The model under review builds one solid part; all positions refer to its coordinate system, in mm. A direction names the side the tool comes from. Round coordinates to 2 decimals unless told otherwise and drop trailing zeros. Write each loop counter-clockwise with the first axis right and the second up, starting at its lowest first coordinate (ties: lowest second). Pieces come first, ordered by that corner, then holes. Notation, with made-up numbers: (5, 73.5) -> (22, 73.5) arc R23 ccw to (22, 103.5) -> close; hole circle Ø2 at (6.25, 1.25). An arc over 180 degrees is marked (long way). Return JSON: item names as keys, results as strings. Group by question number.
1. Take a section at B-B, the plane z = 19. Write out the cut boundary in (x, y), then the cut area to 3 significant figures.
2. Tool access review of faces 1 (the cylindrical face through (-56.8, -57.29, 48.99)), 2 (the flat face through (-24, 0, 12)), 3 (the cylindrical face through (-56.209, -40.367, 111.653)): name each direction out of +Z, -Z, +X, -X, +Y, -Y from which nothing blocks a thin tool from reaching the whole face with its end or side.
3. Take a section at D-D, the plane x = -21.5. Write out the cut boundary in (y, z).
4. Take a section at A-A, the plane y = -46. Write out the cut boundary in (x, z).
5. Mouldability with a two-part tool opening along Y and no side actions: class faces 4 (the cylindrical face through (10.583, -19.163, 6.858)), 5 (the flat face through (-24, -82.55, 12)), 6 (the flat face through (114.516, -41, 6)) as pulls with the +Y half, pulls with the -Y half, needs draft (parallel to the pull), parting line crosses it, or undercut.
6. Take a section at C-C, the plane y = -66. Write out the cut boundary in (x, z), then the cut area to 3 significant figures.
7. For line 1 along X through (y, z) = (-20.5, 75); line 2 along Z through (x, y) = (-34.5, -64.5); line 3 along Z through (x, y) = (-44.5, -33), list the stretches that pass through material, from the lowest coordinate up. Write a range as from..to.
8. Clearance check with flat-ended pins moving along their axes: P1, Ø5, axis at y = -45, z = 27.5, coming from the -X side; P2, Ø4, axis at y = -49.5, z = 37, coming from the +X side; P3, Ø4, axis at y = -25.5, z = 70.5, coming from the +X side. State where each tip first meets the part, or that it passes through.
from build123d import *

# Parameters (mm, degrees)
F1_DEPTH = 82.55
F2_R     = 17.4625
F3_DEPTH = 25.4
F5_DEPTH = 25.4
F6_DEPTH = 37.9726117289
F7_R     = 20.6375
F8_DEPTH = 37.9716117289


with BuildPart() as f1:
    # F0 (on Front) → F1 (new body)
    with BuildSketch(Plane.XZ):
        Polygon((-74.6513270113, 141.1331224257), (-75.983799994, 0), (114.516200006, 0), (114.516200006, 12.7), (-37.8770081944, 14.1387822587), (-36.6780229788, 141.1331224257), align=None)
    extrude(amount=F1_DEPTH)

    # F2 (on face) → F3 (cut)
    with BuildSketch(Plane(origin=(0.1300999203, 0, 13.7799476787), x_dir=(0.9999554344, 0, -0.0094408285), z_dir=(0.0094408285, 0, 0.9999554344))):
        with Locations((12.7911979997, -36.4772640169)):
            Circle(F2_R)
        with Locations((88.9911979997, -36.4772640169)):
            Circle(F2_R)
    extrude(amount=-F3_DEPTH, mode=Mode.SUBTRACT)

    # F5 (cut): a face of the model
    f5_faces = [f1.faces().sort_by_distance(p)[0] for p in [
        (-55.6646749951, -41.275, 141.1331224257),
    ]]
    extrude(f5_faces, amount=-F5_DEPTH, mode=Mode.SUBTRACT)

    # F4 (on face) → F6 (cut, through all)
    with BuildSketch(Plane(origin=(-75.9770276155, 0, 0.7173180531), x_dir=(0, -1, 0), z_dir=(-0.9999554344, 0, 0.0094408285))):
        with BuildLine():
            ThreePointArc((0, 69.852356173), (41.275, 111.127356173), (82.55, 69.852356173))
            Line((82.55, 69.852356173), (82.55, 140.4220623681))
            Line((82.55, 140.4220623681), (0, 140.4220623681))
            Line((0, 140.4220623681), (0, 69.852356173))
        make_face()
    extrude(amount=-F6_DEPTH, mode=Mode.SUBTRACT)

    # F7 (on face) → F8 (cut, through all)
    with BuildSketch(Plane(origin=(-75.9770276155, 0, 0.7173180531), x_dir=(0, -1, 0), z_dir=(-0.9999554344, 0, 0.0094408285))):
        with Locations((38.2229980028, 56.3510982116)):
            Circle(F7_R)
    extrude(amount=-F8_DEPTH, mode=Mode.SUBTRACT)


solid = f1.part
Output:
{
 "1": {"outline": "(-75.8, -82.55) -> (-37.83, -82.55) -> (-37.83, 0) -> (-75.8, 0) -> close", "area": "3,130 mm^2"},
 "2": {"face 1": "none", "face 2": "+Z, -Z, +X, -X, +Y", "face 3": "+Z, +X"},
 "3": {"outline": "(-82.55, 0) -> (0, 0) -> (0, 13.98) -> (-82.55, 13.98) -> close"},
 "4": {"outline": "(-75.98, 0) -> (-1.85, 0) -> (-1.72, 13.8) -> (-37.88, 14.14) -> (-37.66, 37.59) -> (-75.63, 37.95) -> close; (-75.26, 76.18) -> (-37.29, 75.82) -> (-36.96, 111.21) -> (-74.93, 111.57) -> close; (27.43, 0) -> (74.36, 0) -> (74.48, 13.08) -> (27.56, 13.52) -> close; (103.63, 0) -> (114.52, 0) -> (114.52, 12.7) -> (103.75, 12.8) -> close"},
 "5": {"face 4": "undercut", "face 5": "pulls with the -Y half", "face 6": "needs draft"},
 "6": {"outline": "(-75.98, 0) -> (114.52, 0) -> (114.52, 12.7) -> (-37.88, 14.14) -> (-37.04, 103.26) -> (-75.01, 103.62) -> close", "area": "5,970 mm^2"},
 "7": {"line 1": "x = -75.28..-37.3", "line 2": "z = 0..14.11", "line 3": "z = 0..36.81, 76.74..110.71"},
 "8": {"P1": "stops at x = -75.75", "P2": "stops at x = -37.64", "P3": "stops at x = -37.33"}
}
